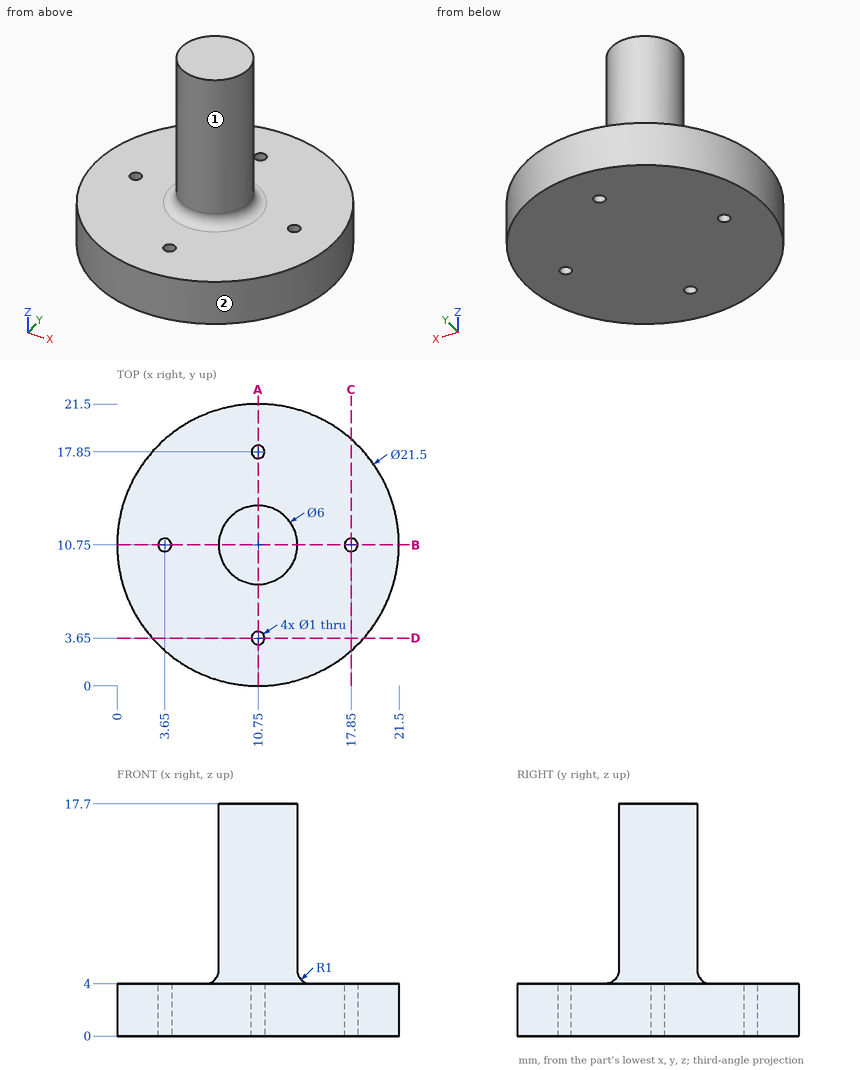
Job drawing, mm, ordinate dimensions from the low corner. One solid piece. A direction names the side the tool comes from. Round coordinates to 2 decimals unless told otherwise and drop trailing zeros. Order: outer loops, then holes, each group sorted by start corner. A loop starts at its lowest first (then second) coordinate and runs counter-clockwise, first axis right, second up. Notation, with made-up numbers: (-11.75, 9) - (8.25, 9) arc R18 ccw to (8.25, 41) - close; hole circle Ø5 at (-35.75, 1). An arc over 180 degrees is marked (long way). Use CSV: the item, a comma, the result in double quotes. Start each with the question number.
1) Tool access for the marked faces 1 and 2: list every direction of +Z, -Z, +X, -X, +Y, -Y with a clear straight run to the whole face (end or side of a thin tool).
2) Pin check, flat tips, straight feed: pin 1 Ø2 at (x, z) = (10, 14) entering from -Y; pin 2 Ø5 at (y, z) = (18.5, 3.5) entering from +X; pin 3 Ø2 at (y, z) = (13.5, 9.5) entering from -X. Stop position of each tip, or through.
3) Saw through at A-A (x = 10.75). List the corners of the cut face in (y, z).
4) Wall check: L1, parallel to Y at x = 10.75, z = 1.05; L2, parallel to Y at x = 17.85, z = 1.15; L3, parallel to Z at x = 9.5, y = 4.5. Give the ranges that are in metal, low to high. Write a range as [from, to].
5) Saw through at C-C (x = 17.85). List the corners of the cut face in (y, z), and give its area (3 significant figures).
Values follow:
1,face 1,"+Z"
1,face 2,"+Z, -Z"
2,pin 1,"stops at y = 7.75"
2,pin 2,"stops at x = 20.13"
2,pin 3,"stops at x = 8.31"
3,outline,"(0, 0) - (3.15, 0) - (3.15, 4) - (0, 4) - close; (4.15, 0) - (17.35, 0) - (17.35, 4) - (14.75, 4) arc R1 cw to (13.75, 5) - (13.75, 17.7) - (7.75, 17.7) - (7.75, 5) arc R1 cw to (6.75, 4) - (4.15, 4) - close; (18.35, 0) - (21.5, 0) - (21.5, 4) - (18.35, 4) - close"
4,L1,"y = [0, 3.15], [4.15, 17.35], [18.35, 21.5]"
4,L2,"y = [2.68, 10.25], [11.25, 18.82]"
4,L3,"z = [0, 4]"
5,outline,"(2.68, 0) - (10.25, 0) - (10.25, 4) - (2.68, 4) - close; (11.25, 0) - (18.82, 0) - (18.82, 4) - (11.25, 4) - close"
5,area,"60.6 mm2"
